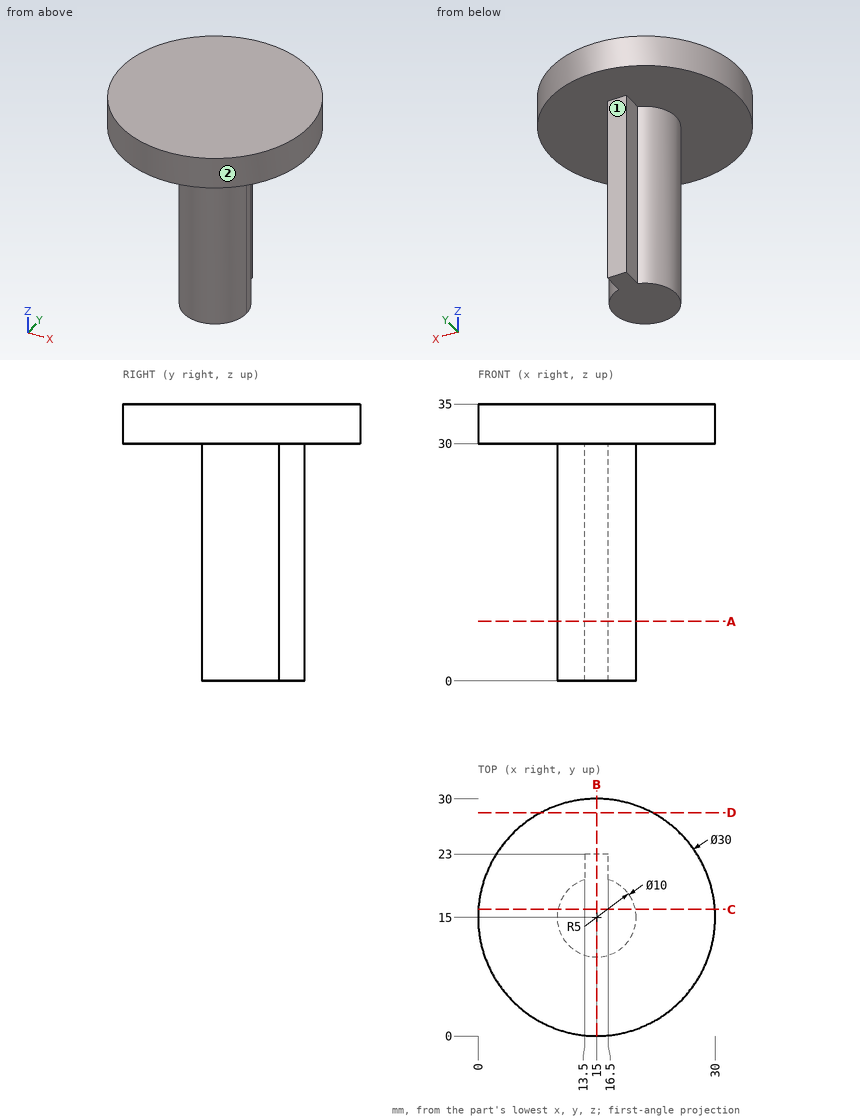
Geometry: see drawing. Coordinates: mm, zero at the bounding-box minimum. A direction names the side the tool comes from. Round coordinates to 2 decimals unless told otherwise and drop trailing zeros. Write each loop counter-clockwise with the first axis right and the second up, starting at its lowest first coordinate (ties: lowest second). Pieces come first, ordered by that corner, then holes.
Item 1: Section query C-C (y = 16). Return loops of the section in (x, z), plus the area to 3 significant figures.
Item 2: Pin query (flat end, axial travel): P1, Ø2, axis at y = 13.5, z = 17, coming from the -X side; P2, Ø1.5, axis at x = 15.5, z = 17.5, coming from the +Y side; P3, Ø2.5, axis at y = 22, z = 16.5, coming from the -X side. Return the tip coordinate at first contact, or that it passes through.
Item 3: Material intervals for L1, parallel to Z at x = 2, y = 21.75; L2, parallel to Y at x = 14.75, z = 7.5; L3, parallel to Y at x = 16, z = 6.5, sorted ascending.
Item 4: Section query B-B (x = 15). Return loops of the section in (y, z), plus the area to 3 significant figures.
Item 5: Section query A-A (z = 7.5). Return loops of the section in (x, y).
Item 6: Section query D-D (y = 28.25). Return loops of the section in (x, z), plus the area to 3 significant figures.
Item 7: Set-up query: the marked faces 1 and 2. Return all of +Z, -Z, +X, -X, +Y, -Y with unobstructed straight access to the full face (end or side cutting, diameter ignored); none if empty.
Completed:
1. outline: (0.03, 30) - (10.1, 30) - (10.1, 0) - (19.9, 0) - (19.9, 30) - (29.97, 30) - (29.97, 35) - (0.03, 35) - close
1. area: 444 mm2
2. P1: stops at x = 10.03
2. P2: stops at y = 23
2. P3: stops at x = 13.5
3. L1: z = 30 to 35
3. L2: y = 10.01 to 23
3. L3: y = 10.1 to 23
4. outline: (0, 30) - (10, 30) - (10, 0) - (23, 0) - (23, 30) - (30, 30) - (30, 35) - (0, 35) - close
4. area: 540 mm2
5. outline: (13.5, 19.77) arc R5 ccw (long way) to (16.5, 19.77) - (16.5, 23) - (13.5, 23) - close
6. outline: (7.97, 30) - (22.03, 30) - (22.03, 35) - (7.97, 35) - close
6. area: 70.3 mm2
7. face 1: -Z, +X, -X, +Y
7. face 2: +Z, -Z
